The listing builds one solid part. Answer for the finished solid, in the listing's coordinates (mm). Coordinates: 2 decimals unless noted, no trailing zeros. Write each loop counter-clockwise with the first axis right and the second up, starting at its lowest first coordinate (ties: lowest second). Pieces come first, ordered by that corner, then holes. Notation, with made-up numbers: M 85,49 L 130,49 A24 cw 130,64 Z; hole C -3.75,-6 d4. An arc over 180 degrees is marked long. Answer as CSV lines item,"result".
```python
from build123d import *

# Parameters (mm, degrees)
SKETCH1_R           = 6
BOSS_EXTRUDE1_DEPTH = 6
SKETCH2_R           = 0.875
SKETCH4_R           = 3.000001976
CUT_EXTRUDE1_DEPTH  = 8


with BuildPart() as part:
    # Sketch1 → Boss-Extrude1 (new body)
    with BuildSketch(Plane(origin=(0, 0, 0), x_dir=(1, 0, 0), z_dir=(0, 1, 0))):
        Circle(SKETCH1_R)
    extrude(amount=BOSS_EXTRUDE1_DEPTH)

    # Sketch2 → Cut-Revolve1 (revolve, cut)
    with BuildSketch(Plane.XY):
        with Locations((6, 2)):
            Circle(SKETCH2_R)
    revolve(axis=Axis((0, 0, 0), (0, 1, 0)), mode=Mode.SUBTRACT)

    # Sketch4 → Cut-Extrude1 (cut)
    with BuildSketch(Plane(origin=(0, 6, 0), x_dir=(1, 0, 0), z_dir=(0, 1, 0))):
        Circle(SKETCH4_R)
    extrude(amount=-CUT_EXTRUDE1_DEPTH, mode=Mode.SUBTRACT)


solid = part.part
```
Q1. Find section C-C (y = 3.25). Give the vertices of the cut face in (x, z), and give its area (3 significant figures).
Output:
outline,"C 0,0 d12; hole C 0,0 d6"
area,"84.8 mm2"
Q2. The mould has two halves that part along Z. Classify faces 1 (the cylindrical face through (2.77, 3.04, 1.15)), 2 (the flat face through (-3, 0, 1)), 3 (the cylindrical face through (-6, 4, 0)): pulls with the +Z half, pulls with the -Z half, needs draft (parallel to the pull), parting line crosses it, or undercut.
Output:
face 1,"undercut"
face 2,"needs draft"
face 3,"parting line crosses it"
Q3. Flat-ended cylindrical pins translate along their axes: pin 1 Ø1.5 at (y, z) = (1.5, 2.5) entering from +X; pin 2 Ø1 at (y, z) = (2.5, -1) entering from -X; pin 3 Ø3 at (x, y) = (3, 1.5) entering from +Z. Find the tip coordinate at first contact, or state that the pin passes through.
Output:
pin 1,"x = 5.71"
pin 2,"x = -5.96"
pin 3,"z = 5.8"
Q4. Straight lines are drawn through the part: line 1 (X direction, y = 3.6, z = 0); line 2 (Z direction, x = -1, y = 5.3). For each, find the intervals that lie inside material, in ascending order.
Output:
line 1,"-6 to -3, 3 to 6"
line 2,"-5.92 to -2.83, 2.83 to 5.92"
Q5. Find section A-A (z = 0). Give the vertices of the cut face in (x, y) (3 decimals).
Output:
outline,"M -6,0 L -3,0 L -3,6 L -6,6 L -6,2.875 A0.875 cw -6,1.125 Z; M 3,0 L 6,0 L 6,1.125 A0.875 cw 6,2.875 L 6,6 L 3,6 Z"
Q6. Find section B-B (x = 0). Give the vertices of the cut face in (y, z) (3 decimals), and give its area (3 significant figures).
Output:
outline,"M 0,-6 L 1.125,-6 A0.875 cw 2.875,-6 L 6,-6 L 6,-3 L 0,-3 Z; M 0,3 L 6,3 L 6,6 L 2.875,6 A0.875 cw 1.125,6 L 0,6 Z"
area,"33.6 mm2"
Q7. Find section D-D (y = 1.45). Give the vertices of the cut face in (x, z).
Output:
outline,"C 0,0 d10.64; hole C 0,0 d6"
